Could you check a few things on this drawing? It's one solid part, dimensions in mm from its lowest x, y, z. Give positions to 0.01 mm unless a question says otherwise; leave off trailing zeros. Loops run counter-clockwise (first coordinate to the right, second up) from the corner with the lowest first, then second, coordinate; pieces in that order, holes last. Notation, with made-up numbers: (-39, -36.75) - (10, -36.75) arc R16 ccw to (10, -22.75) - close; hole circle Ø6 at (66.5, -36.75). An arc over 180 degrees is marked (long way). Write item = value, one per line.
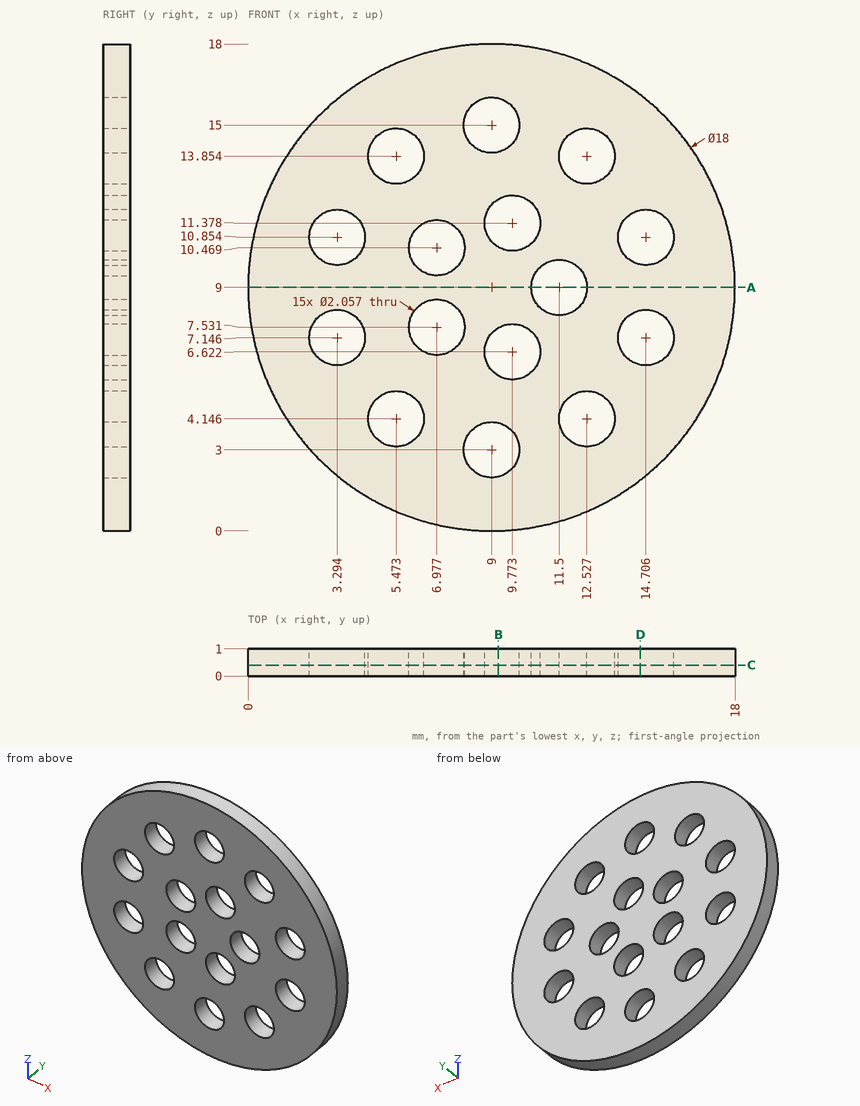
Q1. Imagine slicing it at A-A, the plane z = 9. Write out the boundary of the cut face in (x, y).
Output:
outline = (0, 0) - (10.47, 0) - (10.47, 1) - (0, 1) - close; (12.53, 0) - (18, 0) - (18, 1) - (12.53, 1) - close
Q2. I need wall thicknesses on L1, parallel to X at y = 0.8, z = 3.5 (1 decimal); L2, parallel to Z at x = 13, y = 0.3; L3, parallel to Z at x = 7.25, y = 0.7. Which ranges of each line are inside material? Lowest first, please.
Output:
L1 = 1.9 to 4.7, 6.3 to 8.1, 9.9 to 11.7, 13.3 to 16.1
L2 = 0.94 to 3.23, 5.06 to 12.94, 14.77 to 17.06
L3 = 0.17 to 6.54, 8.52 to 9.48, 11.46 to 17.83
Q3. For pin 1 (1.6 mm diameter, centred on x = 12.53, z = 4.15, fed in from -Y), with a flat end and sliding along its axis, tell me the tip position at first contact or that it passes through.
Output:
pin_1 = through
Q4. Imagine slicing it at D-D, the plane x = 14.5. Write out the boundary of the cut face in (y, z).
Output:
outline = (0, 1.88) - (1, 1.88) - (1, 6.14) - (0, 6.14) - close; (0, 8.15) - (1, 8.15) - (1, 9.85) - (0, 9.85) - close; (0, 11.86) - (1, 11.86) - (1, 16.12) - (0, 16.12) - close
Q5. Imagine slicing it at B-B, the plane x = 9.25. Write out the boundary of the cut face in (y, z).
Output:
outline = (0, 0) - (1, 0) - (1, 2) - (0, 2) - close; (0, 4) - (1, 4) - (1, 5.74) - (0, 5.74) - close; (0, 7.51) - (1, 7.51) - (1, 10.49) - (0, 10.49) - close; (0, 12.26) - (1, 12.26) - (1, 14) - (0, 14) - close; (0, 16) - (1, 16) - (1, 18) - (0, 18) - close
Q6. Imagine slicing it at C-C, the plane y = 0.4. Give the number of separate pieces and of enclosed holes in the cut face.
Output:
separate_pieces = 1
enclosed_holes = 15
